Here's the drawing with two shaded views (mm, measured from the low corner). I have some questions. Give positions to 0.01 mm unless a question says otherwise; leave off trailing zeros. Write each loop counter-clockwise with the first axis right and the second up, starting at its lowest first coordinate (ties: lowest second). Pieces come first, ordered by that corner, then holes. Notation, with made-up numbers: M -21,53.5 L 24,53.5 A21 cw 24,89.5 Z; hole C -29,-35 d8. An arc over 180 degrees is marked long. Use one line per item in the form item = value.
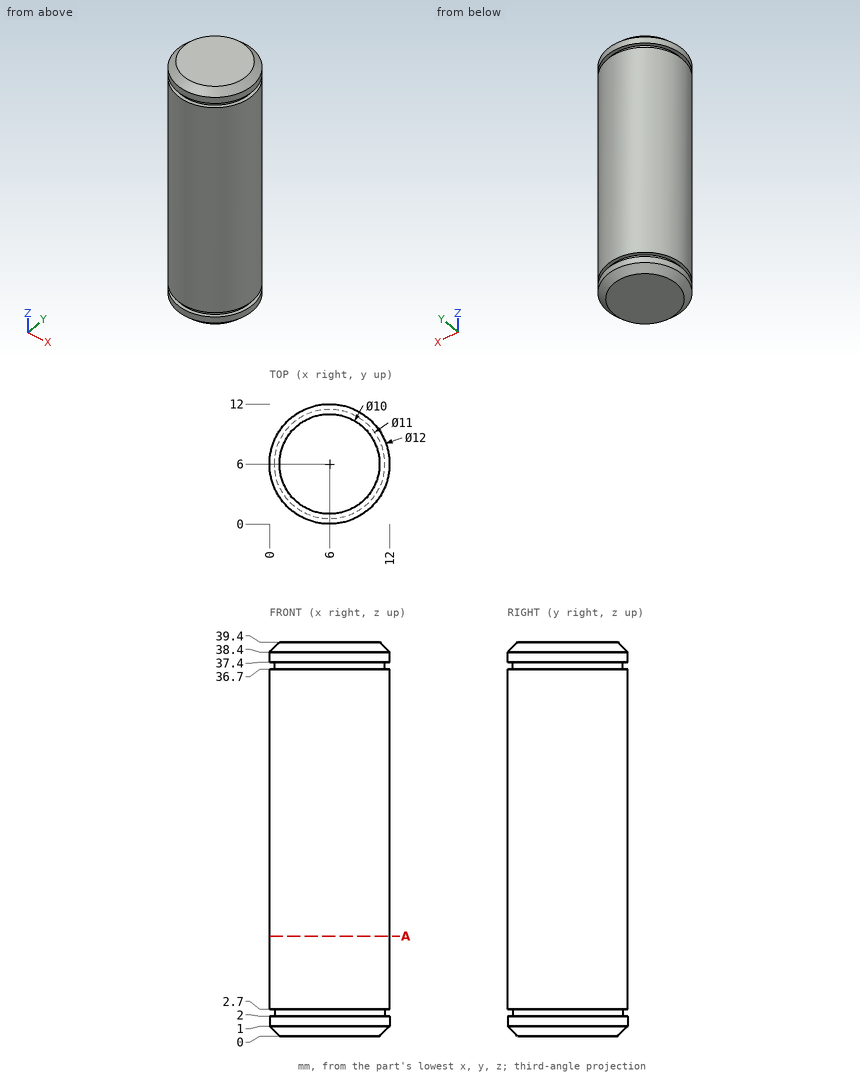
1) I want a section at A-A, the plane z = 10. Please give me the cut outline in (x, y), plus the area to 3 significant figures.
Checked values:
outline = C 6,6 d12
area = 113 mm2
2) If I drill on L1, parallel to Z at x = 0.5, y = 4.5; L2, parallel to Y at x = 5.75, z = 33; L3, parallel to X at y = 2.5, z = 18, over which ranges is the centre line in solid material (lowest first)?
Checked values:
L1 = 0.7 to 2, 2.7 to 36.7, 37.4 to 38.7
L2 = 0.01 to 11.99
L3 = 1.13 to 10.87
3) For pin 1 Ø1.5 at (x, z) = (8.5, 24.5) entering from -Y; pin 2 Ø1.5 at (x, z) = (10.5, 9.5) entering from +Y; pin 3 Ø4 at (y, z) = (2.5, 34) entering from -X, each with a flat end and sliding along its axis, tell me the tip position at first contact or that it passes through.
Checked values:
pin_1 = 0.26
pin_2 = 10.68
pin_3 = 0.19
